from build123d import *

# Parameters (mm, degrees)
SKETCH1_W           = 55
SKETCH1_H           = 75
BOSS_EXTRUDE1_DEPTH = 1.6
SKETCH2_R           = 3.7
BOSS_EXTRUDE2_DEPTH = 12.5


with BuildPart() as part:
    # Sketch1 → Boss-Extrude1 (new body)
    with BuildSketch(Plane(origin=(0, 0, 0), x_dir=(1, 0, 0), z_dir=(0, 1, 0))):
        Rectangle(SKETCH1_W, SKETCH1_H)
    extrude(amount=BOSS_EXTRUDE1_DEPTH)

    # Sketch2 → Boss-Extrude2 (add)
    with BuildSketch(Plane(origin=(0, 1.6, 0), x_dir=(1, 0, 0), z_dir=(0, 1, 0))):
        with Locations(Location((-2.8, -32.4, 0), (0, 0, 270))):
            Circle(SKETCH2_R)
        with Locations(Location((-21.3, -13.8, 0), (0, 0, 270))):
            Circle(SKETCH2_R)
        with Locations(Location((-21.3, 13.8, 0), (0, 0, 270))):
            Circle(SKETCH2_R)
        with Locations(Location((-2.8, 31.2, 0), (0, 0, 270))):
            Circle(SKETCH2_R)
        with Locations(Location((21.3, 13.8, 0), (0, 0, 270))):
            Circle(SKETCH2_R)
        with Locations(Location((21.3, -13.8, 0), (0, 0, 270))):
            Circle(SKETCH2_R)
    extrude(amount=BOSS_EXTRUDE2_DEPTH)


solid = part.part
Design review of the part built by this model. Coordinates are the model's own, in mm. A direction names the side the tool comes from. Coordinates: 2 decimals unless noted, no trailing zeros. Loops run counter-clockwise (first coordinate to the right, second up) from the corner with the lowest first, then second, coordinate; pieces in that order, holes last.
Item 1: Add section D-D (z = -31.2). Write out the cut boundary in (x, y), and give its area (4 significant figures).
Completed:
outline: (-27.5, 0) - (27.5, 0) - (27.5, 1.6) - (0.9, 1.6) - (0.9, 14.1) - (-6.5, 14.1) - (-6.5, 1.6) - (-27.5, 1.6) - close
area: 180.5 mm2
Item 2: Wall thickness on L1, parallel to Y at x = -2, z = 6; L2, parallel to Z at x = -20.5, y = 6.5; L3, parallel to X at y = 7, z = 15: over which ranges is each line inside the solid? List them lowest first.
Completed:
L1: y = 0 to 1.6
L2: z = -17.41 to -10.19, 10.19 to 17.41
L3: x = -24.8 to -17.8, 17.8 to 24.8
Item 3: Add section C-C (x = -2.8). Write out the cut boundary in (y, z), and give its area (3 significant figures).
Completed:
outline: (0, -37.5) - (1.6, -37.5) - (1.6, -34.9) - (14.1, -34.9) - (14.1, -27.5) - (1.6, -27.5) - (1.6, 28.7) - (14.1, 28.7) - (14.1, 36.1) - (1.6, 36.1) - (1.6, 37.5) - (0, 37.5) - close
area: 305 mm2
Item 4: Add section A-A (y = 12). Write out the cut boundary in (x, z), and give its area (3 significant figures).
Completed:
outline: circle Ø7.4 at (-21.3, -13.8); circle Ø7.4 at (-21.3, 13.8); circle Ø7.4 at (-2.8, -31.2); circle Ø7.4 at (-2.8, 32.4); circle Ø7.4 at (21.3, -13.8); circle Ø7.4 at (21.3, 13.8)
area: 258 mm2
Item 5: Add section B-B (z = -13.8). Write out the cut boundary in (x, y).
Completed:
outline: (-27.5, 0) - (27.5, 0) - (27.5, 1.6) - (25, 1.6) - (25, 14.1) - (17.6, 14.1) - (17.6, 1.6) - (-17.6, 1.6) - (-17.6, 14.1) - (-25, 14.1) - (-25, 1.6) - (-27.5, 1.6) - close
Item 6: Clearance check with flat-ended pins moving along their axes: pin 1 (4 mm diameter, centred on y = 5, z = 11.5, fed in from -X); pin 2 (1 mm diameter, centred on x = -22, y = 9.5, fed in from -Z); pin 3 (1 mm diameter, centred on x = -19.5, y = 5, fed in from -Z). State where each tip first meets the part, or that it passes through.
Completed:
pin 1: stops at x = -24.99
pin 2: stops at z = -17.49
pin 3: stops at z = -17.26
Item 7: For faces 4 (the cylindrical face through (-18.8, 7.76, 11.07)), 5 (the flat face through (-21, 14.1, -14)), list the 3-axis set-ups (+Z, -Z, +X, -X, +Y, -Y) from which the entire face can be reached by the end or side of a thin tool; tool diameter is ignored.
Completed:
face 4: +Y
face 5: +Z, -Z, +X, -X, +Y
Item 8: Draft analysis for pull direction X (two halves, no side actions). For faces 1 (the flat face through (0, 1, -37.5)), 2 (the flat face through (-27.5, 1, 1)), 3 (the cylindrical face through (-18.18, 7.76, -11.81)), state which applies: pulls with the +X half, pulls with the -X half, needs draft (parallel to the pull), parting line crosses it, or undercut.
Completed:
face 1: needs draft
face 2: pulls with the -X half
face 3: undercut
